Input: dimensioned drawing with shaded views. Units: mm. Origin: part minimum x, y, z. A direction names the side the tool comes from. Round coordinates to 2 decimals unless told otherwise and drop trailing zeros. Order: outer loops, then holes, each group sorted by start corner. A loop starts at its lowest first (then second) coordinate and runs counter-clockwise, first axis right, second up. Notation, with made-up numbers: M 53,-31 L 68,-31 A35 cw 68,6 Z; hole C 85,71.5 d10. An arc over 180 degrees is marked long. One line per question, with ' | ' between items.
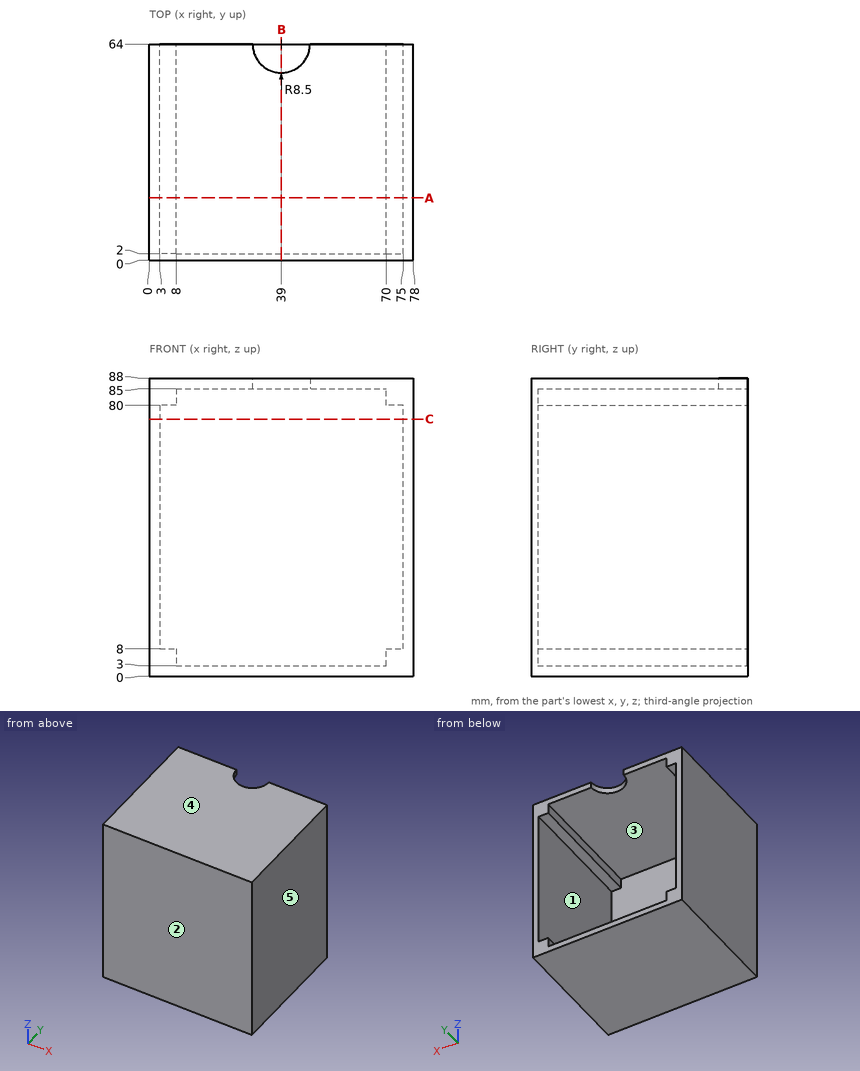
Item 1: Access query for the marked faces 1 and 2. Directions: +Z, -Z, +X, -X, +Y, -Y. A direction counts if a zero-diameter tool reaches every point of the face in a straight line with its end or side. Return the directions, or none.
Report:
face 1: +Y | face 2: +Z, -Z, +X, -X, -Y
Item 2: First-contact query: pin 1 (12 mm diameter, centred on x = 58.5, z = 69, fed in from +Y). Flat tip, straight axial feed; report the tip coordinate or a pass-through.
Report:
pin 1: y = 2
Item 3: Mould query, pull axis X, two halves, no side actions, for the marked faces 3, 4 and 5. Classes: +X half, -X half, draft (parallel to the pull), parting line (faces both ways), or undercut.
Report:
face 3: undercut | face 4: draft | face 5: +X half
Item 4: Section query C-C, the plane z = 76. Return loops of the section in (x, y).
Report:
outline: M 0,0 L 78,0 L 78,64 L 75,64 L 75,2 L 3,2 L 3,64 L 0,64 Z
Item 5: Section query A-A, the plane y = 18.5. Return loops of the section in (x, z).
Report:
outline: M 0,0 L 78,0 L 78,88 L 0,88 Z; hole M 3,8 L 8,8 L 8,3 L 70,3 L 70,8 L 75,8 L 75,80 L 70,80 L 70,85 L 8,85 L 8,80 L 3,80 Z
Item 6: Section query B-B, the plane x = 39. Return loops of the section in (y, z).
Report:
outline: M 0,0 L 64,0 L 64,3 L 2,3 L 2,85 L 55.5,85 L 55.5,88 L 0,88 Z
Item 7: Line query: line 1 along X through (y, z) = (15, 8.5); line 2 along Z through (x, y) = (23, 48); line 3 along X through (y, z) = (30, 81). Output: solid intervals per line, ascending. Write a range as from..to.
Report:
line 1: 0..3, 75..78 | line 2: 0..3, 85..88 | line 3: 0..8, 70..78
